```python
from build123d import *

# Parameters (mm, degrees)
SKETCH1_W           = 20
SKETCH1_H           = 40
SKETCH1_W_2         = 4
SKETCH1_H_2         = 2
BOSS_EXTRUDE1_DEPTH = 2
BOSS_EXTRUDE2_DEPTH = 2
SKETCH3_R           = 2.5
CUT_EXTRUDE1_DEPTH  = 2


with BuildPart() as part:
    # Sketch1 → Boss-Extrude1 (new body)
    with BuildSketch(Plane(origin=(0, 0, 0), x_dir=(1, 0, 0), z_dir=(0, 1, 0))):
        Polygon((0, 0), (5, 0), (5, -2), (9, -2), (9, 0), (12.5, 0), (12.5, 2), (11.4, 2), (11.4, 4.3), (12.5, 4.3), (12.5, 6), (15.5, 6), (15.5, 4.3), (16.6, 4.3), (16.6, 2), (15.5, 2), (15.5, 0), (19, 0), (19, -2), (23, -2), (23, 0), (28, 0), (28, 66), (0, 66), align=None)
        with Locations((14, 33)):
            Rectangle(SKETCH1_W, SKETCH1_H, mode=Mode.SUBTRACT)
        with Locations((7, 64)):
            Rectangle(SKETCH1_W_2, SKETCH1_H_2, mode=Mode.SUBTRACT)
        with Locations((21, 64)):
            Rectangle(SKETCH1_W_2, SKETCH1_H_2, mode=Mode.SUBTRACT)
        with Locations((14, 64)):
            Rectangle(SKETCH1_W_2, SKETCH1_H_2, mode=Mode.SUBTRACT)
    extrude(amount=BOSS_EXTRUDE1_DEPTH)

    # Sketch2 → Boss-Extrude2 (add)
    with BuildSketch(Plane(origin=(0, 2, 0), x_dir=(1, 0, 0), z_dir=(0, 1, 0))):
        with BuildLine():
            Line((0, 66), (28, 66))
            ThreePointArc((28, 66), (34.819271185, 129.864214399), (70.378490249, 183.349560802))
            ThreePointArc((70.378490249, 183.349560802), (70.223472253, 188.82876401), (64.776007814, 189.43772177))
            ThreePointArc((64.776007814, 189.43772177), (17.177564343, 135.700793296), (0, 66))
        make_face()
    extrude(amount=-BOSS_EXTRUDE2_DEPTH)

    # Sketch3 → Cut-Extrude1 (cut)
    with BuildSketch(Plane(origin=(0, 2, 0), x_dir=(1, 0, 0), z_dir=(0, 1, 0))):
        with Locations(Location((44.359461926, 163, 0), (0, 0, 270))):
            Circle(SKETCH3_R)
    extrude(amount=-CUT_EXTRUDE1_DEPTH, mode=Mode.SUBTRACT)


solid = part.part
```
Work out the finished part from the listing and answer in its coordinate system (mm). Coordinates: 2 decimals unless noted, no trailing zeros. Write each loop counter-clockwise with the first axis right and the second up, starting at its lowest first coordinate (ties: lowest second). Pieces come first, ordered by that corner, then holes. Notation, with made-up numbers: (62.25, 59) - (104.25, 59) arc R17 ccw to (104.25, 83) - close; hole circle Ø9 at (-22.75, 31). An arc over 180 degrees is marked (long way). Answer as a JSON object with one key per item and string values.
Q1. Find section D-D (z = -99.5). Write down the section's boundary in (x, y).
Results list:
{"outline": "(3.79, 0) - (27.68, 0) - (27.68, 2) - (3.79, 2) - close"}
Q2. Consider L1, parallel to Z at x = 13.5, y = 1.6; L2, parallel to X at y = 0.8, z = -24; L3, parallel to X at y = 1.45, z = -163. Determine where each line is inside the solid, lowest interval first. Write a range as from..to.
Results list:
{"L1": "z = -128.19..-65, -63..-53, -13..-6", "L2": "x = 0..4, 24..28", "L3": "x = 35.58..41.86, 46.86..52.31"}
Q3. Find section B-B (x = 38). Write down the section's boundary in (y, z).
Results list:
{"outline": "(0, -165.78) - (2, -165.78) - (2, -137.86) - (0, -137.86) - close"}
Q4. For a pull along Z with two mould halves and no side action, classify faces 1 (the cylindrical face through (45.11, 1.014, -160.615)), 2 (the cylindrical face through (17.652, 1.014, -136.598)), 3 (the flat face through (22, 0, -95)) as pulls with the +Z half, pulls with the -Z half, needs draft (parallel to the pull), parting line crosses it, or undercut.
Results list:
{"face 1": "undercut", "face 2": "pulls with the -Z half", "face 3": "needs draft"}
Q5. Find section C-C (y = 0.9). State how many separate pieces and enclosed holes the cut face has, plus the area to 3 significant figures.
Results list:
{"separate pieces": "1", "enclosed holes": "5", "area": "3,540 mm^2"}
Q6. Given pin 1 Ø0.5 at (x, y) = (12, 1) entering from +Z; pin 2 Ø1 at (y, z) = (1, -64) entering from +X; pin 3 Ø1 at (x, y) = (14, 1) entering from +Z, each flat-ended and moving along its own axis, determine where each tip first touches the part or whether it passes through.
Results list:
{"pin 1": "stops at z = 0", "pin 2": "stops at x = 28", "pin 3": "stops at z = -6"}
Q7. Find section A-A (z = -163). Write down the section's boundary in (x, y).
Results list:
{"outline": "(35.58, 0) - (41.86, 0) - (41.86, 2) - (35.58, 2) - close; (46.86, 0) - (52.31, 0) - (52.31, 2) - (46.86, 2) - close"}
